```python
from build123d import *

# Parameters (mm, degrees)
ESQUISSE1_W                  = 80
ESQUISSE1_H                  = 20
BOSS_EXTRU_1_DEPTH           = 5
CONG_1_R                     = 4
ENL_V_MAT_EXTRU_1_DEPTH      = 83.613558209
ENL_V_START                  = -5
ENL_V_MAT_EXTRU_2_DEPTH      = 5
ESQUISSE11_W                 = 13.611032385
ESQUISSE11_H                 = 17.64061434
BOSS_EXTRU_8_DEPTH           = 5
ENL_V_MAT_EXTRU_3_DEPTH      = 83.613558336
ENL_V_MAT_EXTRU_3_DEPTH_BACK = 83.613558336
ESQUISSE13_R                 = 3
ENL_V_MAT_EXTRU_4_DEPTH      = 33


# Read off the part's stored shape, not the designer's step: Enlèv. mat.-Extru.2
with BuildPart() as part:
    # Esquisse1 → Boss.-Extru.1 (new body)
    with BuildSketch(Plane.XY):
        with Locations((40, -10)):
            Rectangle(ESQUISSE1_W, ESQUISSE1_H)
    extrude(amount=BOSS_EXTRU_1_DEPTH)

    # Congé1
    cong_1_edges = [part.edges().sort_by_distance(p)[0] for p in [
        (0, 0, 2.5),
        (80, 0, 2.5),
        (80, -20, 2.5),
        (0, -20, 2.5),
    ]]
    fillet(cong_1_edges, radius=CONG_1_R)

    # Esquisse2 → Enlèv. mat.-Extru.1 (cut, through all)
    with BuildSketch(Plane.XY.offset(5)):
        Polygon((28.410040172, -2.300084773), (30.410040172, -2.300084773), (24.995829866, -18.113699025), (22.995829866, -18.113699025), align=None)
        Polygon((9.298142424, -2.198086037), (16.298142424, -2.198086037), (10.914062948, -18.113699025), (3.914062948, -18.113699025), align=None)
        Polygon((18.309829725, -2.300084773), (22.309829725, -2.300084773), (16.902589817, -18.093340154), (12.902589817, -18.093340154), align=None)
        Polygon((23.808061727, -2.300084773), (26.808061727, -2.300084773), (21.404325417, -18.111661936), (18.404325417, -18.111661936), align=None)
        Polygon((31.786127586, -2.300084773), (33.786127586, -2.300084773), (28.371917279, -18.113699025), (26.371917279, -18.113699025), align=None)
    extrude(amount=-ENL_V_MAT_EXTRU_1_DEPTH, mode=Mode.SUBTRACT)

    # Enlèv. mat.-Extru.2 outline → Enlèv. mat.-Extru.2 (cut)
    # profile 1 of 3: a face of its own
    with BuildSketch(Plane.XY.offset(5).offset(ENL_V_START)):
        with BuildLine():
            add(Edge.make_bspline(
                [(75.686567024, -16.611023442), (75.678643784, -16.704663886), (75.663447013, -16.884266233), (75.563839443, -17.132408637), (75.415616385, -17.347383223), (75.204262037, -17.518269705), (74.945020643, -17.657920052), (74.629763147, -17.753299102), (74.263391467, -17.817731699), (74.000846179, -17.830167685), (73.861085096, -17.83678775)],
                knots=[0, 0, 0, 0, 0.114098337, 0.218840581, 0.322174175, 0.429434412, 0.547100708, 0.679564678, 0.829422238, 1, 1, 1, 1], degree=3))
            Line((75.686567024, -16.611023442), (75.686567024, -9.411486545))
            Line((75.686567024, -9.411486545), (69.882470639, -9.411486545))
            Line((69.882470639, -9.411486545), (69.882470639, -11.283775701))
            Line((69.882470639, -11.283775701), (72.316446542, -11.283775701))
            Line((72.316446542, -11.283775701), (72.316446542, -15.777269677))
            Line((72.316446542, -15.777269677), (67.822952566, -15.777269677))
            Line((67.822952566, -15.777269677), (67.822952566, -4.356305822))
            Line((67.822952566, -4.356305822), (72.316446542, -4.356305822))
            Line((72.316446542, -4.356305822), (72.316446542, -6.977510641))
            Line((72.316446542, -6.977510641), (75.686567024, -6.977510641))
            Line((75.686567024, -6.977510641), (75.686567024, -3.522552057))
            add(Edge.make_bspline(
                [(73.861085096, -2.29678775), (74.000846179, -2.303407815), (74.263391467, -2.3158438), (74.629763147, -2.380276397), (74.945020643, -2.475655447), (75.204262037, -2.615305794), (75.415616385, -2.786192276), (75.563839443, -3.001166862), (75.663447013, -3.249309266), (75.678643784, -3.428911613), (75.686567024, -3.522552057)],
                knots=[0, 0, 0, 0, 0.170577762, 0.320435322, 0.452899292, 0.570565588, 0.677825825, 0.781159419, 0.885901663, 1, 1, 1, 1], degree=3))
            Line((73.861085096, -2.29678775), (66.322195789, -2.29678775))
            add(Edge.make_bspline(
                [(64.452832084, -3.522552057), (64.460490101, -3.428813179), (64.475207603, -3.248661832), (64.578900626, -3.001012416), (64.72992953, -2.785012839), (64.947387079, -2.615412784), (65.212124175, -2.475706721), (65.534969931, -2.379572165), (65.910264022, -2.316247539), (66.179534857, -2.303527098), (66.322195789, -2.29678775)],
                knots=[0, 0, 0, 0, 0.112348161, 0.215915455, 0.318343111, 0.425762474, 0.543690884, 0.676356302, 0.828532073, 1, 1, 1, 1], degree=3))
            Line((64.452832084, -3.522552057), (64.452832084, -16.611023442))
            add(Edge.make_bspline(
                [(66.278314012, -17.83678775), (66.138552929, -17.830167685), (65.876007642, -17.817731699), (65.509635961, -17.753299102), (65.194378466, -17.657920052), (64.935137072, -17.518269705), (64.723782723, -17.347383223), (64.575559665, -17.132408637), (64.475952096, -16.884266233), (64.460755324, -16.704663886), (64.452832084, -16.611023442)],
                knots=[0, 0, 0, 0, 0.170577762, 0.320435322, 0.452899292, 0.570565588, 0.677825825, 0.781159419, 0.885901663, 1, 1, 1, 1], degree=3))
            Line((66.278314012, -17.83678775), (73.861085096, -17.83678775))
        make_face()
    # profile 2 of 3: a face of its own
    with BuildSketch(Plane.XY.offset(5).offset(ENL_V_START)):
        with BuildLine():
            add(Edge.make_bspline(
                [(59.247868229, -10.142849497), (59.250113416, -10.031576234), (59.255029992, -9.787906808), (59.301768342, -9.394005261), (59.364432817, -8.9400039), (59.423938248, -8.619443962), (59.455575307, -8.4490129)],
                knots=[0, 0, 0, 0, 0.195301478, 0.427676852, 0.695714808, 1, 1, 1, 1], degree=3))
            Line((59.247868229, -10.142849497), (59.247868229, -17.83678775))
            Line((59.247868229, -17.83678775), (62.617988711, -17.83678775))
            Line((62.617988711, -17.83678775), (62.617988711, -2.29678775))
            Line((62.617988711, -2.29678775), (59.481904374, -2.29678775))
            Line((59.481904374, -2.29678775), (55.68759338, -10.836181575))
            add(Edge.make_bspline(
                [(55.596904374, -11.538290009), (55.59815665, -11.492405908), (55.600881716, -11.392557927), (55.62162629, -11.229918497), (55.645376833, -11.040932864), (55.672949182, -10.907206292), (55.68759338, -10.836181575)],
                knots=[0, 0, 0, 0, 0.19413449, 0.422454333, 0.693254547, 1, 1, 1, 1], degree=3))
            add(Edge.make_bspline(
                [(55.506215368, -10.836181575), (55.516865461, -10.868148772), (55.54346006, -10.947974815), (55.561126156, -11.099283482), (55.582536457, -11.300899182), (55.59176432, -11.45336457), (55.596904374, -11.538290009)],
                knots=[0, 0, 0, 0, 0.142095852, 0.354830918, 0.640631437, 1, 1, 1, 1], degree=3))
            Line((55.506215368, -10.836181575), (51.711904374, -2.29678775))
            Line((51.711904374, -2.29678775), (48.575820036, -2.29678775))
            Line((48.575820036, -2.29678775), (48.575820036, -17.83678775))
            Line((48.575820036, -17.83678775), (51.945940518, -17.83678775))
            Line((51.945940518, -17.83678775), (51.945940518, -10.142849497))
            add(Edge.make_bspline(
                [(51.741158892, -8.4490129), (51.77262663, -8.62239324), (51.831532725, -8.946952903), (51.895555168, -9.402629403), (51.938009232, -9.793916754), (51.94345609, -10.033548389), (51.945940518, -10.142849497)],
                knots=[0, 0, 0, 0, 0.309420385, 0.579220093, 0.808073296, 1, 1, 1, 1], degree=3))
            Line((51.741158892, -8.4490129), (54.728045187, -16.338956424))
            Line((54.728045187, -16.338956424), (56.480390819, -16.338956424))
            Line((56.480390819, -16.338956424), (59.455575307, -8.4490129))
        make_face()
    # profile 3 of 3: a face of its own
    with BuildSketch(Plane.XY.offset(5).offset(ENL_V_START)):
        Polygon((44.119771843, -17.83678775), (47.489892325, -17.83678775), (43.019801964, -2.29678775), (39.439048952, -2.29678775), (34.945554976, -17.795831424), (34.945554976, -17.83678775), (38.315675458, -17.83678775), (39.023634795, -15.028354015), (43.41766341, -15.028354015), align=None)
        Polygon((41.217723651, -5.921422539), (42.923262054, -12.968835942), (39.488781633, -12.968835942), align=None, mode=Mode.SUBTRACT)
    extrude(amount=ENL_V_MAT_EXTRU_2_DEPTH, mode=Mode.SUBTRACT)

    # Esquisse11 → Boss.-Extru.8 (add)
    with BuildSketch(Plane.XY.offset(5)):
        with Locations((41.097921838, -10.121676789)):
            Rectangle(ESQUISSE11_W, ESQUISSE11_H)
    extrude(amount=-BOSS_EXTRU_8_DEPTH)

    # Esquisse12 → Enlèv. mat.-Extru.3 (cut, two sides: drawn at the far end of the back side and taken through both)
    with BuildSketch(Plane.XY.offset(5).offset(-ENL_V_MAT_EXTRU_3_DEPTH_BACK)):
        Polygon((35.786127586, -2.300084773), (42.786127586, -2.300084773), (48.111179633, -17.834694794), (46.111179633, -17.834694794), (44.102998893, -11.969278829), (35.786127586, -11.969278829), (37.115967439, -10.077108111), (43.455164056, -10.077108111), (41.446983316, -4.211692145), (37.138004335, -4.211692145), (32.518467193, -17.83678775), (30.518467193, -17.83678775), align=None)
    extrude(amount=ENL_V_MAT_EXTRU_3_DEPTH + ENL_V_MAT_EXTRU_3_DEPTH_BACK, mode=Mode.SUBTRACT)

    # Esquisse13 → Enlèv. mat.-Extru.4 (cut)
    with BuildSketch(Plane.XY.offset(5)):
        with Locations((4.24401363, -4.167068495)):
            Circle(ESQUISSE13_R)
    extrude(amount=-ENL_V_MAT_EXTRU_4_DEPTH, mode=Mode.SUBTRACT)


solid = part.part
```
The listing builds one solid part. Answer for the finished solid, in the listing's coordinates (mm). A direction names the side the tool comes from. Round coordinates to 2 decimals unless told otherwise and drop trailing zeros. Order: outer loops, then holes, each group sorted by start corner. A loop starts at its lowest first (then second) coordinate and runs counter-clockwise, first axis right, second up. Notation, with made-up numbers: (78.5, -4) -> (114.5, -4) arc R24 ccw to (114.5, 7) -> close; hole circle Ø2 at (16, 33). An arc over 180 degrees is marked (long way). Answer as CSV lines item,"result".
Q1. Given pin 1 (9.5 mm diameter, centred on x = 4.24, y = -4.17, fed in from -Z), flat-ended and moving along its own axis, determine where the tip first touches the part or whether it passes through.
Computed values:
pin 1,"stops at z = 0"
Q2. A cutting plane is placed at B-B on y = -13.75. Give the number of separate pieces and of enclosed holes in the cut face, plus the area to 3 significant figures.
Computed values:
separate pieces,"13"
enclosed holes,"0"
area,"204 mm^2"
Q3. Consider line 1 (Y direction, x = 37.5, z = 3.35); line 2 (Y direction, x = 49.5, z = 1.15); line 3 (X direction, y = -2.25, z = 3.75). Determine where each line is inside the solid, lowest interval first. Write a range as from..to.
Computed values:
line 1,"y = -20..-11.97, -10.08..-4.21, -2.3..0"
line 2,"y = -20..-17.84, -2.3..0"
line 3,"x = 0.4..1.94, 6.55..9.28, 16.28..79.6"
Q4. A cutting plane is placed at A-A on x = 73. Determine the outline of the cut face in (y, z).
Computed values:
outline,"(-20, 0) -> (-17.84, 0) -> (-17.84, 5) -> (-20, 5) -> close; (-9.41, 0) -> (-6.98, 0) -> (-6.98, 5) -> (-9.41, 5) -> close; (-2.3, 0) -> (0, 0) -> (0, 5) -> (-2.3, 5) -> close"
Q5. Which of the six approach directions +Z, -Z, +X, -X, +Y, -Y give full straight-line access (tool end or side, diameter ignored) to faces 4 (the flat face through (29.04, -10.32, 2.54)), 5 (the flat face through (39, -20, 2))?
Computed values:
face 4,"+Z, -Z"
face 5,"+Z, -Z, +X, -X, -Y"
Q6. For a pull along X with two mould halves and no side action, classify faces 1 (the flat face through (39.4, -9.9, 0)), 2 (the flat face through (0, -10, 2)), 3 (the flat face through (45.41, -9.96, 2.47)) as +X half, -X half, draft (parallel to the pull), parting line (faces both ways), or undercut.
Computed values:
face 1,"draft"
face 2,"-X half"
face 3,"undercut"
Q7. A cutting plane is placed at C-C on x = 19.5. Determine the outline of the cut face in (y, z).
Computed values:
outline,"(-20, 0) -> (-18.11, 0) -> (-18.11, 5) -> (-20, 5) -> close; (-14.91, 0) -> (-10.51, 0) -> (-10.51, 5) -> (-14.91, 5) -> close; (-2.3, 0) -> (0, 0) -> (0, 5) -> (-2.3, 5) -> close"
